Drawing for the job (mm, zero at the part's lowest x, y, z). A direction names the side the tool comes from. Give positions to 0.01 mm unless a question says otherwise; leave off trailing zeros. Loops run counter-clockwise (first coordinate to the right, second up) from the corner with the lowest first, then second, coordinate; pieces in that order, holes last.
1) 3-axis set-ups, long thin cutter, end or side, ignore diameter. For the marked faces 4 and 5: which of +Z, -Z, +X, -X, +Y, -Y reach the whole face in a straight line?
2) Band-saw the part on A-A on y = 8. List the corners of the cut face in (x, z).
3) Band-saw the part on C-C on x = 47.5. List the corners of the cut face in (y, z).
4) Band-saw the part on B-B on z = 10.75. List the corners of the cut face in (x, y).
5) Wall check: line 1 (Z direction, x = 7, y = 5.25); line 2 (X direction, y = 5.75, z = 3.75); line 3 (Y direction, x = 32.5, z = 5.5). Give the ranges that are in metal, low to high.
6) Two-plate mould, pull along X, no slides. Class the marked faces 1, 2 and 3: +X half, -X half, draft (parallel to the pull), parting line (faces both ways), or undercut.
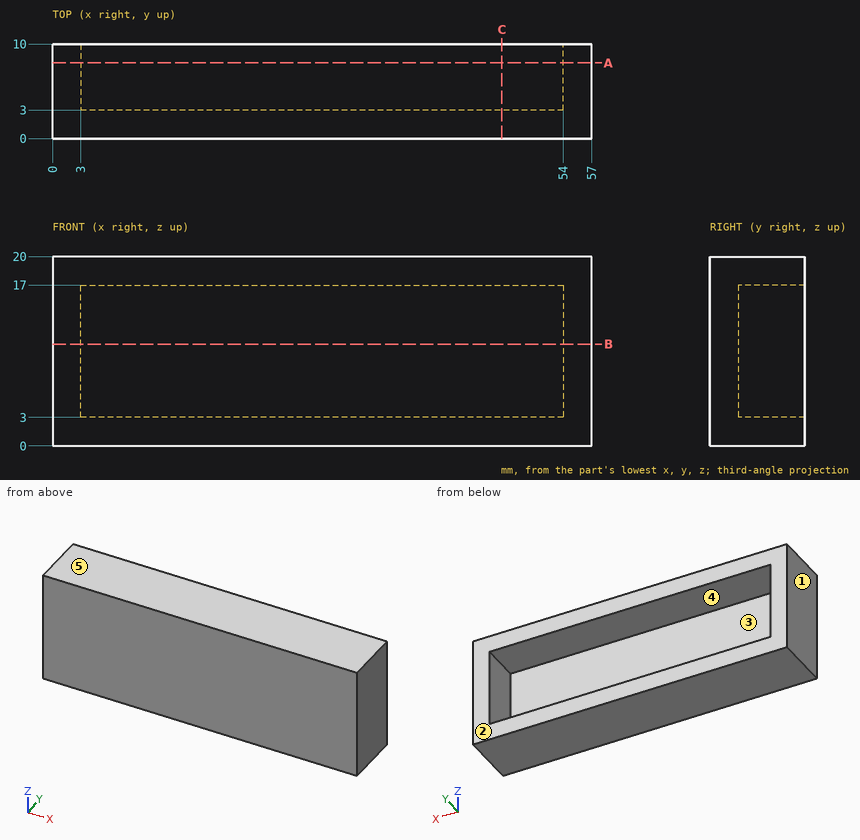
Findings below:
1. face 4: +Y
1. face 5: +Z, +X, -X, +Y, -Y
2. outline: (0, 0) - (57, 0) - (57, 20) - (0, 20) - close; hole (3, 3) - (54, 3) - (54, 17) - (3, 17) - close
3. outline: (0, 0) - (10, 0) - (10, 3) - (3, 3) - (3, 17) - (10, 17) - (10, 20) - (0, 20) - close
4. outline: (0, 0) - (57, 0) - (57, 10) - (54, 10) - (54, 3) - (3, 3) - (3, 10) - (0, 10) - close
5. line 1: z = 0 to 3, 17 to 20
5. line 2: x = 0 to 3, 54 to 57
5. line 3: y = 0 to 3
6. face 1: -X half
6. face 2: draft
6. face 3: undercut
